```python
from build123d import *

# Parameters (mm, degrees)
SKETCH_W        = 50
SKETCH_H        = 30
PAD_DEPTH       = 3
SKETCH001_W     = 20
SKETCH001_H     = 4
PAD001_DEPTH    = 70
SKETCH002_R     = 1.4
POCKET_DEPTH    = 5
CHAMFER_SIZE    = 2
CHAMFER001_SIZE = 2
CHAMFER002_SIZE = 2


with BuildPart() as part:
    # Sketch → Pad (new body)
    with BuildSketch(Plane.XY):
        Rectangle(SKETCH_W, SKETCH_H)
    extrude(amount=PAD_DEPTH)

    # Sketch001 (on Face6 of Pad) → Pad001 (join)
    with BuildSketch(Plane.XY.offset(3)):
        Rectangle(SKETCH001_W, SKETCH001_H)
    extrude(amount=PAD001_DEPTH)

    # Sketch002 (on Face9 of Pad001) → Pocket (cut)
    with BuildSketch(Plane.XZ.offset(2)):
        with Locations((-6, 70)):
            Circle(SKETCH002_R)
        with Locations((6, 70)):
            Circle(SKETCH002_R)
    extrude(amount=-POCKET_DEPTH, mode=Mode.SUBTRACT)

    # Chamfer
    chamfer_edges = [part.edges().sort_by_distance(p)[0] for p in [
        (10, 0, 3),
        (0, -2, 3),
        (0, 2, 3),
        (-10, 0, 3),
    ]]
    chamfer(chamfer_edges, length=CHAMFER_SIZE)

    # Chamfer001
    chamfer001_edges = [part.edges().sort_by_distance(p)[0] for p in [
        (-25, -15, 1.5),
        (-25, 15, 1.5),
        (25, -15, 1.5),
        (25, 15, 1.5),
    ]]
    chamfer(chamfer001_edges, length=CHAMFER001_SIZE)

    # Chamfer002
    chamfer002_edges = [part.edges().sort_by_distance(p)[0] for p in [
        (10, 0, 73),
        (-10, 0, 73),
    ]]
    chamfer(chamfer002_edges, length=CHAMFER002_SIZE)


solid = part.part
```
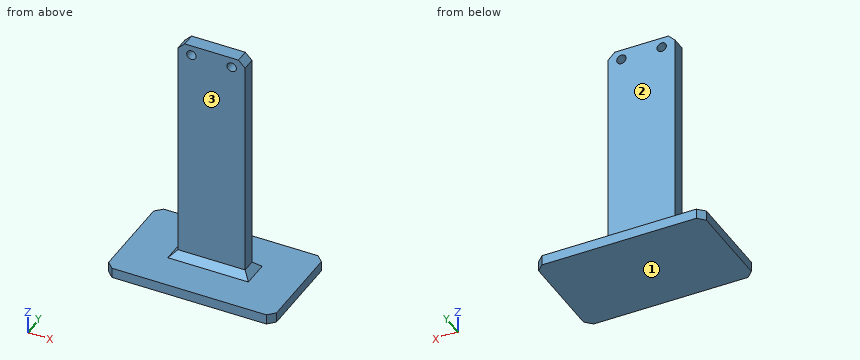
Can you work these out from the model? Positions are in its coordinate system, mm. Face numbers are marked on the shaded views. A direction names the side the tool comes from. Give positions to 0.01 mm unless a question says otherwise; leave off trailing zeros. Order: outer loops, then holes, each group sorted by start corner. A loop starts at its lowest first (then second) coordinate and runs counter-clockwise, first axis right, second up. Notation, with made-up numbers: (61.5, 71) - (107.5, 71) arc R21 cw to (107.5, 86) - close; hole circle Ø11 at (28, 62.5). An arc over 180 degrees is marked (long way). Use a Markdown table: item, result. Add a question column.
Q1. Please list where these lines run through material, in increasing order: line 1 along X through (y, z) = (0.65, 70); line 2 along Z through (x, y) = (-6, -0.35); line 3 along Z through (x, y) = (-16.5, -11.5).
Q2. If we section it at C-C on z = 70: Write out the boundary of the cut face in (x, y).
Q3. I'm going to push flat-ended pins straight in: pin 1 (2 mm diameter, centred on y = 0.5, z = 30.5, fed in from -X); pin 2 (6 mm diameter, centred on x = -6.5, z = 11.5, fed in from -Y); pin 3 (6 mm diameter, centred on x = -3, z = 51.5, fed in from +Y). Where does each tip first touch, or does it pass through?
Q4. If we section it at B-B on y = 1: Write out the boundary of the cut face in (x, z).
Q5. If we section it at D-D on x = -3.5: Write out the boundary of the cut face in (y, z).
Q6. On a 3-axis mill with a long thin cutter (end or side, diameter ignored), from which of +Z, -Z, +X, -X, +Y, -Y can I reach the whole of each face in a straight line? I mean the marked faces 1, 2 and 3. Say none if no direction works.
Q7. If we section it at A-A on x = 6: Write out the boundary of the cut face in (y, z).
Answers follow:
| question | item | result |
|---|---|---|
| 1 | line 1 | x = -10 to -7.4, -4.6 to 4.6, 7.4 to 10 |
| 1 | line 2 | z = 0 to 68.6, 71.4 to 73 |
| 1 | line 3 | z = 0 to 3 |
| 2 | outline | (-10, -2) - (-7.4, -2) - (-7.4, 2) - (-10, 2) - close; (-4.6, -2) - (4.6, -2) - (4.6, 2) - (-4.6, 2) - close; (7.4, -2) - (10, -2) - (10, 2) - (7.4, 2) - close |
| 3 | pin 1 | stops at x = -10 |
| 3 | pin 2 | stops at y = -2 |
| 3 | pin 3 | stops at y = 2 |
| 4 | outline | (-25, 0) - (25, 0) - (25, 3) - (12, 3) - (10, 5) - (10, 71) - (8, 73) - (-8, 73) - (-10, 71) - (-10, 5) - (-12, 3) - (-25, 3) - close; hole circle Ø2.8 at (-6, 70); hole circle Ø2.8 at (6, 70) |
| 5 | outline | (-15, 0) - (15, 0) - (15, 3) - (4, 3) - (2, 5) - (2, 73) - (-2, 73) - (-2, 5) - (-4, 3) - (-15, 3) - close |
| 6 | face 1 | -Z, +X, -X, +Y, -Y |
| 6 | face 2 | +Z, +X, -X, +Y |
| 6 | face 3 | +Z, +X, -X, -Y |
| 7 | outline | (-15, 0) - (15, 0) - (15, 3) - (4, 3) - (2, 5) - (2, 68.6) - (-2, 68.6) - (-2, 5) - (-4, 3) - (-15, 3) - close; (-2, 71.4) - (2, 71.4) - (2, 73) - (-2, 73) - close |
